The listing builds one solid part. Answer for the finished solid, in the listing's coordinates (mm). A direction names the side the tool comes from. Round coordinates to 2 decimals unless told otherwise and drop trailing zeros. Order: outer loops, then holes, each group sorted by start corner. A loop starts at its lowest first (then second) coordinate and runs counter-clockwise, first axis right, second up. Notation, with made-up numbers: (-12, 84) - (15, 84) arc R20 cw to (15, 90) - close; hole circle Ø7 at (73.5, 2.25). An arc over 180 degrees is marked (long way). One line per item, written item: value. Start each with the question number.
1. For a pull along Y with two mould halves and no side action, classify faces 1 (the flat face through (0.3, 72.5, -4.8)), 2 (the flat face through (-2.5, 57, 33)), 3 (the flat face through (-12.547, 60, 12)) as released by +Y, released by -Y, zero draft, split by the parting line, or undercut.
2. Straight lines are drawn through the part: line 1 (X direction, y = 50.25, z = 24); line 2 (X direction, y = 68.75, z = -25); line 3 (X direction, y = 51, z = 7). For each, find the intervals that lie inside material, in ascending order.
3. Section C-C, the plane z = 3.5 is taken. Give the vertices of the cut face in (x, y), then the cut area to 3 significant figures.
4. Section B-B, the plane y = 59.5 is taken. Give the vertices of the cut face in (x, z), then the cut area to 3 significant figures.
5. Section D-D, the plane z = 32.2 is taken. Give the vertices of the cut face in (x, y), then the cut area to 3 significant figures.
6. Flat-ended cylindrical pins translate along their axes: P1, Ø4.5, axis at x = 6.5, z = 27, coming from the -Y side; P2, Ø4, axis at x = 12, z = -20, coming from the -Y side; P3, Ø0.9, axis at y = 57, z = 32, coming from the -X side; P4, Ø3.5, axis at x = -3, y = 62, coming from the +Z side. Find the tip coordinate at first contact, or state that the pin passes through.
7. Section A-A, the plane x = 0 is taken. Count the separate pieces of the cut face and the enclosed holes in it, then the cut area to 3 significant figures.
8. A tool of negligible diameter and unlimited length cuts with its end or side. For faces 4 (the flat face through (15, 60, -17)), 5 (the flat face through (8, 55.25, 24)), 6 (the flat face through (-6.23, 64, 18)), from which of +Z, -Z, +X, -X, +Y, -Y can it reach the whole face along a straight path? Write none if from no direction.
from build123d import *
from OCP.BRepFilletAPI import BRepFilletAPI_MakeChamfer

# Parameters (mm, degrees)
SKETCH4_W                = 12.46
SKETCH4_H                = 17.25
BOSS_EXTRUDE3_DEPTH      = 6
BOSS_EXTRUDE6_DEPTH      = 7.3
BOSS_EXTRUDE6_DEPTH_BACK = 17.25
SKETCH8_R                = 12.546781182
SKETCH8_R_2              = 11.15
BOSS_EXTRUDE4_DEPTH      = 17.25
SKETCH6_R                = 2
CUT_EXTRUDE1_DEPTH       = 5
CHAMFER1_SIZE            = 0.5
CHAMFER1_SIZE_2          = 0.866025404
SKETCH10_W               = 12.46
SKETCH10_H               = 23.7
CUT_EXTRUDE3_DEPTH       = 17.25
CUT_EXTRUDE4_REACH       = 83.955
SKETCH11_W               = 5
SKETCH11_H               = 3
BOSS_EXTRUDE7_START      = -7.3
BOSS_EXTRUDE7_DEPTH      = 7.3
BOSS_EXTRUDE8_DEPTH      = 24.55


with BuildPart() as part:
    # Sketch4 → Boss-Extrude3 (new body)
    with BuildSketch(Plane.XY):
        with Locations((0, 63.875025481)):
            Rectangle(SKETCH4_W, SKETCH4_H)
    extrude(amount=BOSS_EXTRUDE3_DEPTH)



with BuildPart() as body_2:
    # Sketch8 → Boss-Extrude6 (new, two sides: drawn at the far end of the back side and taken through both)
    with BuildSketch(Plane(origin=(0, 55.250025481, 0), x_dir=(-1, 0, 0), z_dir=(0, -1, 0)).offset(-BOSS_EXTRUDE6_DEPTH_BACK)):
        with Locations(Location((0, -23.55, 0), (0, 0, 90))):
            Circle(SKETCH8_R)
        with Locations(Location((0, -23.55, 0), (0, 0, 90))):
            Circle(SKETCH8_R_2, mode=Mode.SUBTRACT)
    extrude(amount=BOSS_EXTRUDE6_DEPTH + BOSS_EXTRUDE6_DEPTH_BACK)


with BuildPart() as part_1:
    add(part.part)

    add(body_2.part)  # Boss-Extrude4 merges body 2
    # Sketch5 → Boss-Extrude4 (add)
    with BuildSketch(Plane(origin=(0, 72.500025481, 0), x_dir=(1, 0, 0), z_dir=(0, 1, 0))):
        with BuildLine():
            Line((12.546781182, -23.55), (12.546781182, 0))
            Line((12.546781182, 0), (6.23, 0))
            Line((6.23, 0), (6.23, -29.7))
            Line((6.23, -29.7), (-6.23, -29.7))
            Line((-6.23, -29.7), (-6.23, 0))
            Line((-6.23, 0), (-12.546781182, 0))
            Line((-12.546781182, 0), (-12.546781182, -23.55))
            ThreePointArc((-12.546781182, -23.55), (0, -36.096781182), (12.546781182, -23.55))
        make_face()
    extrude(amount=-BOSS_EXTRUDE4_DEPTH)

    # Sketch6 → Cut-Extrude1 (cut)
    with BuildSketch(Plane(origin=(0, 72.500025481, 0), x_dir=(1, 0, 0), z_dir=(0, 1, 0))):
        with Locations(Location((0, -3.5, 0), (0, 0, 270))):
            Circle(SKETCH6_R)
        with Locations(Location((0, -32.2, 0), (0, 0, 270))):
            Circle(SKETCH6_R)
    extrude(amount=-CUT_EXTRUDE1_DEPTH, mode=Mode.SUBTRACT)

    # Chamfer1
    chamfer1_edges_1 = [part_1.edges().sort_by_distance(p)[0] for p in [
        (0, 72.500025481, 1.5),
    ]]
    chamfer1_side_1 = [part_1.faces().sort_by_distance(p)[0] for p in [
        (0, 72.500025481, 1.49),
    ]]
    chamfer1_edges_2 = [part_1.edges().sort_by_distance(p)[0] for p in [
        (0, 72.500025481, 30.2),
    ]]
    chamfer1_side_2 = [part_1.faces().sort_by_distance(p)[0] for p in [
        (0, 72.500025481, 30.19),
    ]]
    chamfer1 = BRepFilletAPI_MakeChamfer(part_1.part.solid().wrapped)
    for e in chamfer1_edges_1:
        chamfer1.Add(CHAMFER1_SIZE - 0.0001, CHAMFER1_SIZE_2 - 0.0001, e.wrapped, chamfer1_side_1[0].wrapped)
    for e in chamfer1_edges_2:
        chamfer1.Add(CHAMFER1_SIZE - 0.0001, CHAMFER1_SIZE_2 - 0.0001, e.wrapped, chamfer1_side_2[0].wrapped)
    add(Compound.cast(chamfer1.Shape()), mode=Mode.REPLACE)  # a hair under: the kernel refuses the full size

    # Sketch10 → Cut-Extrude3 (cut)
    with BuildSketch(Plane(origin=(0, 72.500025481, 0), x_dir=(1, 0, 0), z_dir=(0, 1, 0))):
        with Locations((0, -17.85)):
            Rectangle(SKETCH10_W, SKETCH10_H)
    extrude(amount=-CUT_EXTRUDE3_DEPTH, mode=Mode.SUBTRACT)

    # Sketch11 → Cut-Extrude4 (cut, up to next)
    with BuildSketch(Plane.XY.offset(36.096781182), mode=Mode.PRIVATE) as cut_extrude4_sk1:
        with Locations((0, 56.750025481)):
            Rectangle(SKETCH11_W, SKETCH11_H)
    cut_extrude4_tool1 = extrude(cut_extrude4_sk1.sketch, amount=-CUT_EXTRUDE4_REACH, mode=Mode.PRIVATE) & part_1.part
    add(cut_extrude4_tool1.solids().sort_by_distance((0, 56.750025, 36.096781))[0], mode=Mode.SUBTRACT)

    # Sketch13 → Boss-Extrude7 (add)
    with BuildSketch(Plane.XZ.offset(-47.950025481).offset(BOSS_EXTRUDE7_START)):
        with BuildLine():
            Line((-12.546781182, 23.55), (-12.546781182, 0))
            Line((-12.546781182, 0), (12.546781182, 0))
            Line((12.546781182, 0), (12.546781182, 23.55))
            ThreePointArc((12.546781182, 23.55), (0, 11.003218818), (-12.546781182, 23.55))
        make_face()
    extrude(amount=BOSS_EXTRUDE7_DEPTH)

    # Sketch14 → Boss-Extrude8 (add)
    with BuildSketch(Plane(origin=(0, 72.500025481, 0), x_dir=(1, 0, 0), z_dir=(0, 1, 0))):
        Polygon((-25, 0), (-25, 30), (-15, 30), (-15, 5), (15, 5), (15, 30), (25, 30), (25, 0), align=None)
    extrude(amount=-BOSS_EXTRUDE8_DEPTH)


solid = part_1.part
Answer list:
1. face 1: released by +Y
1. face 2: undercut
1. face 3: zero draft
2. line 1: x = -12.54 to -11.14, 11.14 to 12.54
2. line 2: x = -25 to -15, 15 to 25
2. line 3: x = -12.55 to 12.55
3. outline: (-12.55, 47.95) - (12.55, 47.95) - (12.55, 72.5) - (2.5, 72.5) - (2, 71.63) - (2, 67.5) - (-2, 67.5) - (-2, 71.63) - (-2.5, 72.5) - (-12.55, 72.5) - close
3. area: 596 mm²
4. outline: (-25, -30) - (-15, -30) - (-15, -5) - (15, -5) - (15, -30) - (25, -30) - (25, 0) - (12.55, 0) - (12.55, 23.55) arc R12.55 ccw to (-12.55, 23.55) - (-12.55, 0) - (-25, 0) - close; hole (-6.23, 6) - (6.23, 6) - (6.23, 29.7) - (-6.23, 29.7) - close
4. area: 1,290 mm²
5. outline: (-9.09, 47.95) - (-7.04, 47.95) - (-7.04, 55.25) - (-2.5, 55.25) - (-2.5, 58.25) - (2.5, 58.25) - (2.5, 55.25) - (7.04, 55.25) - (7.04, 47.95) - (9.09, 47.95) - (9.09, 72.5) - (2.5, 72.5) - (2, 71.63) - (2, 67.5) - (-2, 67.5) - (-2, 71.63) - (-2.5, 72.5) - (-9.09, 72.5) - close
5. area: 308 mm²
6. P1: stops at y = 55.25
6. P2: passes through
6. P3: stops at x = -9.67
6. P4: stops at z = 36.03
7. separate pieces: 3
7. enclosed holes: 0
7. area: 377 mm²
8. face 4: -Z, +Y, -Y
8. face 5: -Y
8. face 6: +Y
